Answer from the drawing. Dimensions are ordinates in mm from the lowest x, y and z of the part. A direction names the side the tool comes from. Coordinates: 2 decimals unless noted, no trailing zeros. Order: outer loops, then holes, each group sorted by start corner. A loop starts at its lowest first (then second) coordinate and runs counter-clockwise, first axis right, second up. Notation, with made-up numbers: (74, 54) -> (78, 54) arc R19 ccw to (78, 72) -> close; hole circle Ø3 at (67.5, 19.5). An arc over 180 degrees is marked (long way). Answer as a JSON object with one key per item and string values. Group by question number.
1) A tool of negligible diameter and unlimited length cuts with its end or side. For the marked faces 4, 5, 6 and 7, from which of +Z, -Z, +X, -X, +Y, -Y can it reach the whole face along a straight path? Write none if from no direction.
2) Consider L1, parallel to Y at x = 16.95, z = 29; L2, parallel to Z at x = 6.5, y = 8.75; L3, parallel to X at y = 6.5, z = 25. Determine where each line is inside the solid, lowest interval first.
3) Given pin 1 (3 mm diameter, centred on x = 15, y = 9, fed in from -Z); pin 2 (1.7 mm diameter, centred on x = 9.5, y = 2.5, fed in from +Z); pin 3 (2 mm diameter, centred on x = 8, y = 7, fed in from +Z); pin 4 (4 mm diameter, centred on y = 5, z = 6, fed in from -X), each flat-ended and moving along its own axis, determine where each tip first touches the part or whether it passes through.
4) Section C-C on z = 6.5 is taken. Determine the outline of the cut face in (x, y).
5) Section D-D on z = 17.5 is taken. Determine the outline of the cut face in (x, y).
6) Determine the mould class of the marked faces 1, 2 and 3 for opening direction X: released by +X, released by -X, zero draft, split by the parting line, or undercut.
7) Section B-B on x = 5 is taken. Determine the outline of the cut face in (y, z).
8) Section A-A on z = 25.5 is taken. Determine the outline of the cut face in (x, y).
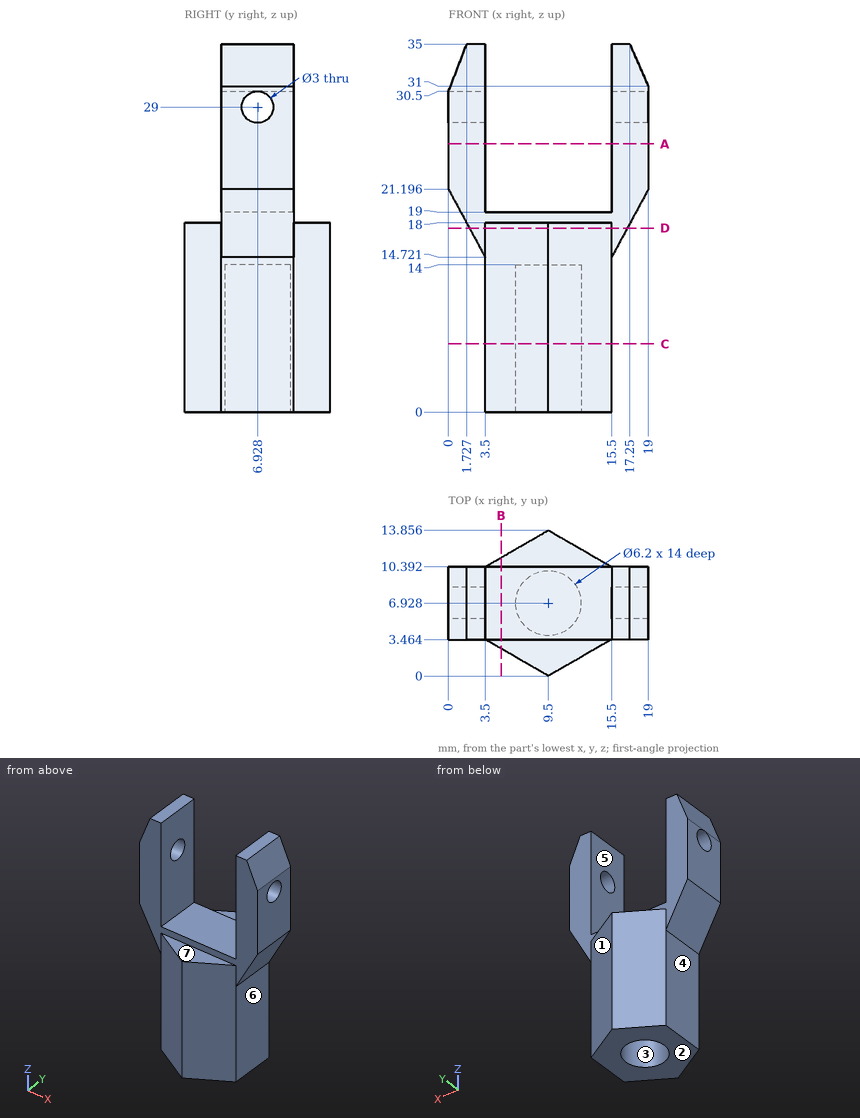
Worked answers:
{
 "1": {"face 4": "-Z, -X, +Y, -Y", "face 5": "+Z, +Y, -Y", "face 6": "-Z, +X, +Y, -Y", "face 7": "+Z, +X, -X, -Y"},
 "2": {"L1": "y = 3.46 to 5.43, 8.43 to 10.39", "L2": "z = 0 to 19", "L3": "x = 0 to 3.5, 15.5 to 19"},
 "3": {"pin 1": "stops at z = 0", "pin 2": "stops at z = 18", "pin 3": "stops at z = 19", "pin 4": "stops at x = 3.5"},
 "4": {"outline": "(3.5, 3.46) -> (9.5, 0) -> (15.5, 3.46) -> (15.5, 10.39) -> (9.5, 13.86) -> (3.5, 10.39) -> close; hole circle Ø6.2 at (9.5, 6.93)"},
 "5": {"outline": "(2, 3.46) -> (3.5, 3.46) -> (9.5, 0) -> (15.5, 3.46) -> (17, 3.46) -> (17, 10.39) -> (15.5, 10.39) -> (9.5, 13.86) -> (3.5, 10.39) -> (2, 10.39) -> close"},
 "6": {"face 1": "released by +X", "face 2": "zero draft", "face 3": "undercut"},
 "7": {"outline": "(2.6, 0) -> (11.26, 0) -> (11.26, 18) -> (10.39, 18) -> (10.39, 19) -> (3.46, 19) -> (3.46, 18) -> (2.6, 18) -> close"},
 "8": {"outline": "(0, 3.46) -> (3.5, 3.46) -> (3.5, 10.39) -> (0, 10.39) -> close; (15.5, 3.46) -> (19, 3.46) -> (19, 10.39) -> (15.5, 10.39) -> close"}
}
